```python
from build123d import *

# Parameters (mm, degrees)
F3_DEPTH = 175.35396


with BuildPart() as f1:
    # F0 (on Front) → F1 (revolve)
    with BuildSketch(Plane.XZ):
        with BuildLine():
            Line((0, 21.537127), (0, 0))
            Line((0, 0), (108.105168, 0))
            Line((108.105168, 0), (108.105168, 20.936103))
            ThreePointArc((108.105168, 20.936103), (106.924834, 24.623521), (103.822632, 26.940109))
            ThreePointArc((103.822632, 26.940109), (94.951811, 39.376777), (103.822632, 51.813444))
            ThreePointArc((103.822632, 51.813444), (106.924834, 54.130032), (108.105168, 57.81745))
            Line((108.105168, 57.81745), (108.105168, 72.403553))
            ThreePointArc((108.105168, 72.403553), (106.245296, 76.893681), (101.755168, 78.753553))
            Line((101.755168, 78.753553), (89.708269, 78.753553))
            Line((89.708269, 78.753553), (3.092389, 26.987858))
            ThreePointArc((3.092389, 26.987858), (0.826942, 24.670549), (0, 21.537127))
        make_face()
    revolve(axis=Axis((0, 0, 17.780939), (0, 0, -1)))

    # F2 (on face) → F3 (cut)
    with BuildSketch(Plane(origin=(0, 0, 0), x_dir=(1, 0, 0), z_dir=(0, 0, -1))):
        Polygon((16.383819, 28.377607), (-16.383819, 28.377607), (-32.767639, 0), (-16.383819, -28.377607), (16.383819, -28.377607), (32.767639, 0), align=None)
    extrude(amount=-F3_DEPTH, mode=Mode.SUBTRACT)


solid = f1.part
```
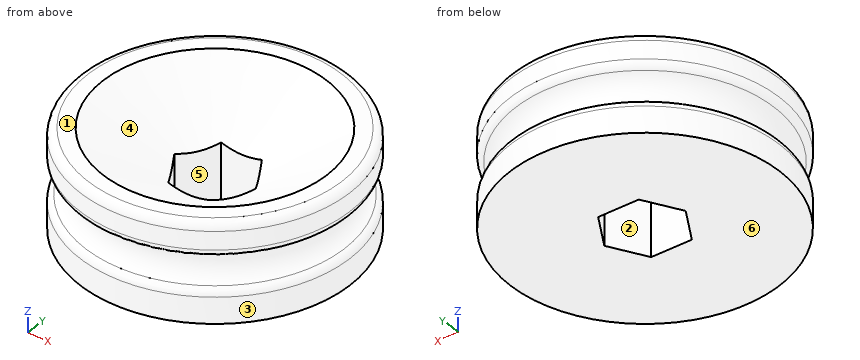
For this review, take the finished solid that the model builds, in its own axes (mm). Face numbers are marked on the shaded views. A direction names the side the tool comes from. Coordinates: 2 decimals unless noted, no trailing zeros. Write each loop counter-clockwise with the first axis right and the second up, starting at its lowest first coordinate (ties: lowest second). Pieces come first, ordered by that corner, then holes.
(1) The part is to be moulded in two halves that separate along X. For the marked faces 1, 2, 3 and 4, say which applies: +X half, -X half, draft (parallel to the pull), parting line (faces both ways), or undercut.
(2) For pin 1 Ø8 at (x, z) = (14.5, 48.5) entering from -Y; pin 2 Ø4 at (x, z) = (-25.5, 58) entering from +Y; pin 3 Ø3 at (y, z) = (-1.5, 24) entering from +X, all flat-tipped, find the tip position at first contact; note any pin that passes through.
(3) Wall thickness on probe 1 along Y at (x, z) = (-30.5, 25); probe 2 along Y at (x, z) = (-8.5, 60.5); probe 3 along X at (y, z) = (-10.5, 48): over which ranges is each line inside the solid? List them lowest first.
(4) Tool access review of the marked faces 5 and 6: name each direction out of +Z, -Z, +X, -X, +Y, -Y from which nothing blocks a thin tool from reaching the whole face with its end or side.
(5) Add section A-A on x = 0. Give the boundary of the cut face in (y, z).
Answer sheet:
1. face 1: draft
1. face 2: undercut
1. face 3: parting line
1. face 4: undercut
2. pin 1: stops at y = -104.25
2. pin 2: stops at y = 105.52
2. pin 3: stops at x = 107.9
3. probe 1: y = -102.18 to -3.93, 3.93 to 102.18
3. probe 2: y = -107.77 to -58.55, 58.55 to 107.77
3. probe 3: x = -97.61 to -36.78, 36.78 to 97.61
4. face 5: +Z, -Z
4. face 6: -Z, +X, -X, +Y, -Y
5. outline: (-108.11, 0) - (-28.38, 0) - (-28.38, 42.1) - (-89.71, 78.75) - (-101.76, 78.75) arc R6.35 ccw to (-108.11, 72.4) - (-108.11, 57.82) arc R6.35 ccw to (-103.82, 51.81) arc R13.15 cw to (-103.82, 26.94) arc R6.35 ccw to (-108.11, 20.94) - close; (28.38, 0) - (108.11, 0) - (108.11, 20.94) arc R6.35 ccw to (103.82, 26.94) arc R13.15 cw to (103.82, 51.81) arc R6.35 ccw to (108.11, 57.82) - (108.11, 72.4) arc R6.35 ccw to (101.76, 78.75) - (89.71, 78.75) - (28.38, 42.1) - close
